Part model, mm, in its own coordinate system. A direction names the side the tool comes from. Give positions to 0.01 mm unless a question says otherwise; leave off trailing zeros. Write each loop counter-clockwise with the first axis right and the second up, starting at its lowest first coordinate (ties: lowest second). Pieces come first, ordered by that corner, then holes. Notation, with made-up numbers: (9, 22) - (51, 22) arc R20 ccw to (51, 36) - close; hole circle Ø11 at (8, -15). An arc over 180 degrees is marked (long way). Answer in a Markdown table with one row per item. Add a question column.
1. Which spindle directions (+Z, -Z, +X, -X, +Y, -Y) get a long thin tool onto all of the face, cutting with end or side? Do faces 4 (the flat face through (-1, 229, -50.8)), 5 (the flat face through (-3, -3, 203.2)), 6 (the cylindrical face through (-10.05, -228.38, -25.76)). Say none if no direction does.
2. Band-saw the part on D-D on y = -236. Write the cut outline in (x, z), plus the area to 3 significant figures.
3. Band-saw the part on A-A on x = 0. Write the cut outline in (y, z).
4. Probe line 1 along Y through (x, z) = (0, -28); line 2 along Z through (x, y) = (-137, 165). List the from-to ranges inside material, lowest first.
5. Band-saw the part on C-C on z = 80. Write the cut outline in (x, y), plus the area to 3 significant figures.
6. Pull direction X, two halves, no side cores. Call faces 1 (the cylindrical face through (-10.05, -228.38, 228.24)), 2 (the cylindrical face through (170.011, -221.722, 103.734)), 3 (the flat face through (-1, -229, 254)): released by +X, released by -X, zero draft, split by the parting line, or undercut.
7. Drop flat-ended pins along their axis: pin 1 Ø6 at (x, y) = (-71.5, 141) entering from -Z; pin 2 Ø1.5 at (y, z) = (132, 147.5) entering from -X; pin 3 Ø2 at (y, z) = (118.5, 218) entering from -X. Give the stop position or say it passes through.
```python
from build123d import *

# Parameters (mm, degrees)
F0_W   = 228.6
F0_H   = 203.2
F0_W_2 = 25.4


with BuildPart() as f1:
    # F0 (on Right) → F1 (revolve)
    with BuildSketch(Plane.YZ):
        with Locations((114.3, 101.6)):
            Rectangle(F0_W, F0_H)
        with Locations((241.3, 101.6)):
            Rectangle(F0_W_2, F0_H)
        Polygon((254, 0), (228.6, 0), (228.6, -50.8), (279.4, -50.8), (279.4, 254), (228.6, 254), (228.6, 203.2), (254, 203.2), align=None)
    revolve(axis=Axis((0, 0, 101.6), (0, 0, 1)))


solid = f1.part
```
Values:
| question | item | result |
|---|---|---|
| 1 | face 4 | -Z, +X, -X, +Y, -Y |
| 1 | face 5 | +Z |
| 1 | face 6 | -Z |
| 2 | outline | (-149.56, -50.8) - (149.56, -50.8) - (149.56, 254) - (-149.56, 254) - close |
| 2 | area | 91,200 mm² |
| 3 | outline | (-279.4, -50.8) - (-228.6, -50.8) - (-228.6, 0) - (228.6, 0) - (228.6, -50.8) - (279.4, -50.8) - (279.4, 254) - (228.6, 254) - (228.6, 203.2) - (-228.6, 203.2) - (-228.6, 254) - (-279.4, 254) - close |
| 4 | line 1 | y = -279.4 to -228.6, 228.6 to 279.4 |
| 4 | line 2 | z = 0 to 203.2 |
| 5 | outline | circle Ø558.8 at (0, 0) |
| 5 | area | 245,000 mm² |
| 6 | face 1 | undercut |
| 6 | face 2 | split by the parting line |
| 6 | face 3 | zero draft |
| 7 | pin 1 | stops at z = 0 |
| 7 | pin 2 | stops at x = -246.65 |
| 7 | pin 3 | stops at x = -253.49 |
